Autodesk Inventor part; units mm, degrees
ref_plane "Work Plane2" through (16, -9.3875, 7) normal (0, 1, 0) x (-1, 0, 0)
ref_plane "YZ Plane" through (0, 0, 0) normal (1, 0, 0) x (0, 1, 0)
ref_plane "XY Plane" through (0, 0, 0) normal (0, 0, 1) x (1, 0, 0)
sketch "Sketch5" plane through (0, 0, 0) normal (1, 0, 0) x (0, 1, 0)
  line L0 (5, 7) -> (-6, 7)
  line L1 (-6, 7) -> (-6, -5)
  line L2 (-6, -5) -> (5, -5)
  line L3 (5, -5) -> (5, 7)
  line L4 (-6, -5) -> (5, -5)
  line L5 (5, -5) -> (5, -7)
  line L6 (5, -7) -> (-6, -7)
  line L7 (-6, -7) -> (-6, -5)
  line L8 (5, 7) -> (-6, 7)
  line L9 (-6, 7) -> (-6, 5)
  line L10 (-6, 5) -> (5, 5)
  line L11 (5, 5) -> (5, 7)
  line L12 (-51.3319, 0) -> (14.3886, 0)
  line L13 (0, -30.178) -> (0, 30.178)
  circle A0 centre (-20.3875, 0) radius 16
  circle A1 centre (-20.3875, 0) radius 21.5557
  line L14 (4, 6) -> (-4.4815, 6)
  line L15 (-4.4815, 6) -> (-4.4815, -6)
  line L16 (-4.4815, -6) -> (4, -6)
  line L17 (4, -6) -> (4, 6)
  circle A2 centre (-20.3875, 0) radius 17
  line L18 (-4.4815, -6) -> (-7.3875, -6)
  line L19 (-7.3875, -6) -> (-7.3875, 6)
  line L20 (-7.3875, 6) -> (-4.4815, 6)
  line L21 (-4.4815, 6) -> (-4.4815, -6)
  line L22 (-6, -7) -> (-9.3875, -7)
  line L23 (-9.3875, -7) -> (-9.3875, 7)
  line L24 (-9.3875, 7) -> (-6, 7)
  line L25 (-6, 7) -> (-6, -7)
  point P0 (0, 0)
  point P1 (0, 7)
  point P2 (-6, 7)
  point P3 (-6, -7)
  point P4 (5, -5)
  point P5 (0.5803, -5)
  point P6 (0.5803, 5)
  point P7 (4, -5)
  point P8 (4, 5)
  point P9 (-4.4815, -6)
  point P10 (-6, 7)
  point P11 (-6, -7)
  point P12 (-4.4815, -6)
  point P13 (-4.4815, 6)
  dimension "d14" = 32
  dimension "d25" = 1
  dimension "d15" = 12
  dimension "d16" = 2
  dimension "d17" = 2
  dimension "d18" = 6
  dimension "d19" = 5
  dimension "d20" = 1
  dimension "d22" = 1
  dimension "d23" = 1
  dimension "d31" = 2
  dimension "d32" = 5
extrude "Extrusion4" add sketch "Sketch5" along normal mid plane 32 contours L3 L10 L17 L14 A1 L0 | L13 L14 A2 L0 | A1 L14 L13 | A2 L20 A0 L0 | L14 A1 L10 L13 | L13 L10 A2 L14 | L14 L17 L10 A1 | A0 L20 L1 | L1 L20 L19 L12 L23 L24 | A2 L10 L15 | L15 L10 A0 L20 | L13 L12 A2 L10 | L10 A1 L12 L13 | A1 L16 L17 L2 L5 L6 | L6 A2 L16 L13 | L13 L16 A1 | L20 A0 L10 L1 | L1 L12 L19 L20 | L15 A0 L10 | L10 A2 L12 A0 L15 | L6 A0 L18 A2 | L13 L2 A2 L12 | L12 A1 L2 L13 | L16 A2 L2 L13 | L13 L2 A1 L16 | A1 L2 L17 L16 | L10 A0 L15 L12 L1 | L12 L19 L18 L7 L22 L23 | L7 L18 A0 | A0 L12 L15 | A2 L2 L15 A0 L12 | L18 A0 L2 L15 | L15 L2 A2 | L12 L15 A0 L2 L1 | L1 L7 L18 L19 L12 | L7 L2 A0 L18 | A0 L15 L12 | L2 A0 L15
extrude "Extrusion5" cut sketch "Sketch5" along normal mid plane 30 contours L14 A1 L10 L13 | L13 L10 A2 L14 | L14 L17 L10 A1 | A2 L10 L15 | L15 L10 A0 L20 | L13 L12 A2 L10 | L10 A1 L12 L13 | L20 A0 L10 L1 | L1 L12 L19 L20 | L15 A0 L10 | L10 A2 L12 A0 L15 | L13 L2 A2 L12 | L12 A1 L2 L13 | L16 A2 L2 L13 | L13 L2 A1 L16 | A1 L2 L17 L16 | L10 A0 L15 L12 L1 | A0 L12 L15 | A2 L2 L15 A0 L12 | L18 A0 L2 L15 | L15 L2 A2 | L12 L15 A0 L2 L1 | L1 L7 L18 L19 L12 | L7 L2 A0 L18 | A0 L15 L12 | L2 A0 L15
ref_plane "Work Plane2" through (16, -9.3875, 7) normal (0, 1, 0) x (-1, 0, 0)
sketch "Sketch9" plane through (16, -9.3875, 7) normal (0, 1, 0) x (-1, 0, 0)
  line L0 (38.4, -7) -> (-6.4, -7)
  line L1 (16, -16.8) -> (16, 2.8)
  point P0 (16, -7)
  point P1 (6, -7)
  point P2 (16, -7)
  point P3 (26, -7)
  dimension "d33" = 20
hole "Hole1" at (10, -9.3875, 0) at (-10, -9.3875, 0) direction (0, 1, 0) diameter 3.5 depth 5
hole "Hole2" at (0, -9.3875, 0) direction (0, 1, 0) diameter 5 depth 1
equation "\"d25\" = d20"
equation "\"d17\" = d16"
equation "\"d22\" = d20"
equation "\"d23\" = d22"
properties part number "Test_Switch_Housing"
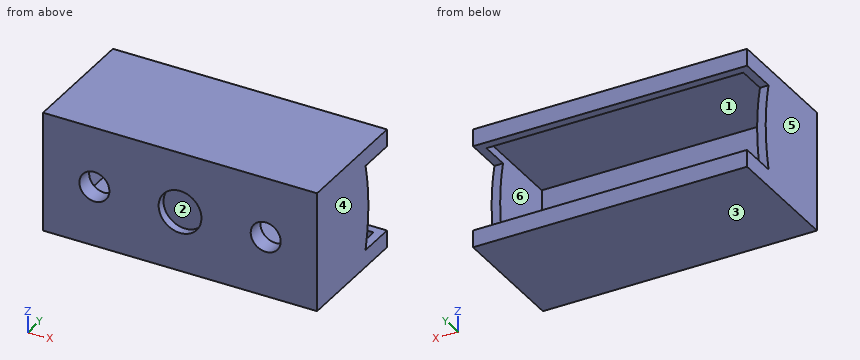
Geometry check sheet. Reference: the model listing, model coordinates, mm. Face numbers are marked on the shaded views. A direction names the side the tool comes from. Give positions to 0.01 mm unless a question says otherwise; leave off trailing zeros. Write each loop counter-clockwise with the first axis right and the second up, starting at its lowest first coordinate (ties: lowest second). Pieces come first, ordered by that corner, then holes.
1) Section check D-D, the plane y = 2. Record the boundary of the cut face in (x, z), and give its area (3 significant figures).
2) Section check A-A, the plane y = -6. Record the boundary of the cut face in (x, z), and give its area (3 significant figures).
3) Section check C-C, the plane z = 0. Record the boundary of the cut face in (x, y).
4) Material ranges on L1, parallel to X at y = -8.8, z = 0; L2, parallel to Z at x = -10, y = -8.4; L3, parallel to Z at x = -2, y = 1.5, recorded low to high.
5) Access from +Z, -Z, +X, -X, +Y, -Y to the whole of each face (thin tool, end or side, straight path). Record for the marked faces 1, 2 and 3.
6) Release check for a two-part mould opening along X. For the marked faces 4, 5 and 6 record: pulls with the +X half, pulls with the -X half, needs draft (parallel to the pull), parting line crosses it, or undercut.
7) Gauge pin test, flat end, axial feed: pin 1 (5 mm diameter, centred on x = 7.5, z = -1.5, fed in from +Y). Record the tip position at first contact, or that the pin passes through.
8) Section check B-B, the plane x = 10. Record the boundary of the cut face in (y, z), and give its area (3 significant figures).
Computed:
1. outline: (-16, -7) - (16, -7) - (16, -5) - (15, -5) - (15, -6) - (-15, -6) - (-15, -5) - (-16, -5) - close; (-16, 5) - (-15, 5) - (-15, 6) - (15, 6) - (15, 5) - (16, 5) - (16, 7) - (-16, 7) - close
1. area: 68.0 mm2
2. outline: (-16, -7) - (16, -7) - (16, 7) - (-16, 7) - close; hole (-15, -6) - (15, -6) - (15, 6) - (-15, 6) - close
2. area: 88.0 mm2
3. outline: (-16, -9.39) - (-11.75, -9.39) - (-11.75, -7.39) - (-15, -7.39) - (-15, 1.17) - (-16, 1.17) - close; (-8.25, -9.39) - (-2.5, -9.39) - (-2.5, -8.39) - (2.5, -8.39) - (2.5, -9.39) - (8.25, -9.39) - (8.25, -7.39) - (-8.25, -7.39) - close; (11.75, -9.39) - (16, -9.39) - (16, 1.17) - (15, 1.17) - (15, -7.39) - (11.75, -7.39) - close
4. L1: x = -16 to -11.75, -8.25 to -2.5, 2.5 to 8.25, 11.75 to 16
4. L2: z = -7 to -1.75, 1.75 to 7
4. L3: z = -7 to -6, 6 to 7
5. face 1: none
5. face 2: -Y
5. face 3: -Z, +X, -X, +Y, -Y
6. face 4: pulls with the +X half
6. face 5: pulls with the -X half
6. face 6: undercut
7. pin 1: stops at y = -7.39
8. outline: (-9.39, -7) - (5, -7) - (5, -5) - (4, -5) - (4, -6) - (-7.39, -6) - (-7.39, -1.75) - (-9.39, -1.75) - close; (-9.39, 1.75) - (-7.39, 1.75) - (-7.39, 6) - (4, 6) - (4, 5) - (5, 5) - (5, 7) - (-9.39, 7) - close
8. area: 47.8 mm2
